The model under review builds one solid part; all positions refer to its coordinate system, in mm. A direction names the side the tool comes from. Round coordinates to 2 decimals unless told otherwise and drop trailing zeros. Loops run counter-clockwise (first coordinate to the right, second up) from the corner with the lowest first, then second, coordinate; pieces in that order, holes last. Notation, with made-up numbers: M 28,-35 L 76,-35 A14 cw 76,-19 Z; hole C 63,60.25 d8. An arc over 180 degrees is marked long. Use a Markdown table: item, result. Add a question column.
```python
from build123d import *

# Parameters (mm, degrees)
SKETCH_1_W          = 106
SKETCH_1_H          = 40
EXTRUDE_1_DEPTH     = 3
CUT_EXTRUDE_1_REACH = 58.727
SKETCH_2_R          = 4.25
SKETCH_2_R_2        = 2.75
CUT_EXTRUDE_2_REACH = 58.727
CUT_EXTRUDE_3_REACH = 58.727
SKETCH_4_W          = 2
SKETCH_4_H          = 4


with BuildPart() as part:
    # 草图1 → 凸台-拉伸1 (new body)
    with BuildSketch(Plane(origin=(0, 0, 0), x_dir=(1, 0, 0), z_dir=(0, 1, 0))):
        Rectangle(SKETCH_1_W, SKETCH_1_H)
    extrude(amount=EXTRUDE_1_DEPTH)

    # 草图2 → 切除-拉伸1 (cut, up to next)
    with BuildSketch(Plane(origin=(0, 3, 0), x_dir=(1, 0, 0), z_dir=(0, 1, 0)), mode=Mode.PRIVATE) as cut_extrude_1_sk1:
        with Locations(Location((-31.5, 0, 0), (0, 0, 270))):
            Circle(SKETCH_2_R)
    cut_extrude_1_tool1 = extrude(cut_extrude_1_sk1.sketch, amount=-CUT_EXTRUDE_1_REACH, mode=Mode.PRIVATE) & part.part
    # 草图2 → 切除-拉伸1 (cut, up to next)
    with BuildSketch(Plane(origin=(0, 3, 0), x_dir=(1, 0, 0), z_dir=(0, 1, 0)), mode=Mode.PRIVATE) as cut_extrude_1_sk2:
        with Locations(Location((31.5, 0, 0), (0, 0, 270))):
            Circle(SKETCH_2_R)
    cut_extrude_1_tool2 = extrude(cut_extrude_1_sk2.sketch, amount=-CUT_EXTRUDE_1_REACH, mode=Mode.PRIVATE) & part.part
    # 草图2 → 切除-拉伸1 (cut, up to next)
    with BuildSketch(Plane(origin=(0, 3, 0), x_dir=(1, 0, 0), z_dir=(0, 1, 0)), mode=Mode.PRIVATE) as cut_extrude_1_sk3:
        with Locations(Location((-47.5, 0, 0), (0, 0, 270))):
            Circle(SKETCH_2_R_2)
    cut_extrude_1_tool3 = extrude(cut_extrude_1_sk3.sketch, amount=-CUT_EXTRUDE_1_REACH, mode=Mode.PRIVATE) & part.part
    # 草图2 → 切除-拉伸1 (cut, up to next)
    with BuildSketch(Plane(origin=(0, 3, 0), x_dir=(1, 0, 0), z_dir=(0, 1, 0)), mode=Mode.PRIVATE) as cut_extrude_1_sk4:
        with Locations(Location((-15.5, 0, 0), (0, 0, 270))):
            Circle(SKETCH_2_R_2)
    cut_extrude_1_tool4 = extrude(cut_extrude_1_sk4.sketch, amount=-CUT_EXTRUDE_1_REACH, mode=Mode.PRIVATE) & part.part
    # 草图2 → 切除-拉伸1 (cut, up to next)
    with BuildSketch(Plane(origin=(0, 3, 0), x_dir=(1, 0, 0), z_dir=(0, 1, 0)), mode=Mode.PRIVATE) as cut_extrude_1_sk5:
        with Locations(Location((15.5, 0, 0), (0, 0, 270))):
            Circle(SKETCH_2_R_2)
    cut_extrude_1_tool5 = extrude(cut_extrude_1_sk5.sketch, amount=-CUT_EXTRUDE_1_REACH, mode=Mode.PRIVATE) & part.part
    # 草图2 → 切除-拉伸1 (cut, up to next)
    with BuildSketch(Plane(origin=(0, 3, 0), x_dir=(1, 0, 0), z_dir=(0, 1, 0)), mode=Mode.PRIVATE) as cut_extrude_1_sk6:
        with Locations(Location((47.5, 0, 0), (0, 0, 270))):
            Circle(SKETCH_2_R_2)
    cut_extrude_1_tool6 = extrude(cut_extrude_1_sk6.sketch, amount=-CUT_EXTRUDE_1_REACH, mode=Mode.PRIVATE) & part.part
    add(cut_extrude_1_tool1.solids().sort_by_distance((-31.5, 3, 0))[0], mode=Mode.SUBTRACT)
    add(cut_extrude_1_tool2.solids().sort_by_distance((31.5, 3, 0))[0], mode=Mode.SUBTRACT)
    add(cut_extrude_1_tool3.solids().sort_by_distance((-47.5, 3, 0))[0], mode=Mode.SUBTRACT)
    add(cut_extrude_1_tool4.solids().sort_by_distance((-15.5, 3, 0))[0], mode=Mode.SUBTRACT)
    add(cut_extrude_1_tool5.solids().sort_by_distance((15.5, 3, 0))[0], mode=Mode.SUBTRACT)
    add(cut_extrude_1_tool6.solids().sort_by_distance((47.5, 3, 0))[0], mode=Mode.SUBTRACT)

    # 草图3 → 切除-拉伸2 (cut, up to next)
    with BuildSketch(Plane(origin=(0, 3, 0), x_dir=(1, 0, 0), z_dir=(0, 1, 0)), mode=Mode.PRIVATE) as cut_extrude_2_sk1:
        Polygon((1.25, 13.25), (10, 13.25), (10, 3.75), (1.25, 3.75), (1.25, -8.75), (-1.25, -8.75), (-1.25, 3.75), (-10, 3.75), (-10, 13.25), (-1.25, 13.25), (-1.25, 17.25), (1.25, 17.25), align=None)
    cut_extrude_2_tool1 = extrude(cut_extrude_2_sk1.sketch, amount=-CUT_EXTRUDE_2_REACH, mode=Mode.PRIVATE) & part.part
    add(cut_extrude_2_tool1.solids().sort_by_distance((0, 3, -7.305405))[0], mode=Mode.SUBTRACT)

    # 草图4 → 切除-拉伸3 (cut, up to next)
    with BuildSketch(Plane(origin=(0, 3, 0), x_dir=(1, 0, 0), z_dir=(0, 1, 0)), mode=Mode.PRIVATE) as cut_extrude_3_sk1:
        with Locations((-3.75, 15.25)):
            Rectangle(SKETCH_4_W, SKETCH_4_H)
    cut_extrude_3_tool1 = extrude(cut_extrude_3_sk1.sketch, amount=-CUT_EXTRUDE_3_REACH, mode=Mode.PRIVATE) & part.part
    # 草图4 → 切除-拉伸3 (cut, up to next)
    with BuildSketch(Plane(origin=(0, 3, 0), x_dir=(1, 0, 0), z_dir=(0, 1, 0)), mode=Mode.PRIVATE) as cut_extrude_3_sk2:
        with Locations((3.75, 15.25)):
            Rectangle(SKETCH_4_W, SKETCH_4_H)
    cut_extrude_3_tool2 = extrude(cut_extrude_3_sk2.sketch, amount=-CUT_EXTRUDE_3_REACH, mode=Mode.PRIVATE) & part.part
    # 草图4 → 切除-拉伸3 (cut, up to next)
    with BuildSketch(Plane(origin=(0, 3, 0), x_dir=(1, 0, 0), z_dir=(0, 1, 0)), mode=Mode.PRIVATE) as cut_extrude_3_sk3:
        with Locations((3.75, -2.5)):
            Rectangle(SKETCH_4_W, SKETCH_4_H)
    cut_extrude_3_tool3 = extrude(cut_extrude_3_sk3.sketch, amount=-CUT_EXTRUDE_3_REACH, mode=Mode.PRIVATE) & part.part
    # 草图4 → 切除-拉伸3 (cut, up to next)
    with BuildSketch(Plane(origin=(0, 3, 0), x_dir=(1, 0, 0), z_dir=(0, 1, 0)), mode=Mode.PRIVATE) as cut_extrude_3_sk4:
        with Locations((-3.75, -2.5)):
            Rectangle(SKETCH_4_W, SKETCH_4_H)
    cut_extrude_3_tool4 = extrude(cut_extrude_3_sk4.sketch, amount=-CUT_EXTRUDE_3_REACH, mode=Mode.PRIVATE) & part.part
    add(cut_extrude_3_tool1.solids().sort_by_distance((-3.75, 3, -15.25))[0], mode=Mode.SUBTRACT)
    add(cut_extrude_3_tool2.solids().sort_by_distance((3.75, 3, -15.25))[0], mode=Mode.SUBTRACT)
    add(cut_extrude_3_tool3.solids().sort_by_distance((3.75, 3, 2.5))[0], mode=Mode.SUBTRACT)
    add(cut_extrude_3_tool4.solids().sort_by_distance((-3.75, 3, 2.5))[0], mode=Mode.SUBTRACT)


solid = part.part
```
(1) Consider section A-A, the plane x = -7.5. Give the boundary of the cut face in (y, z).
(2) Insertion check: pin 1 Ø13.5 at (x, z) = (-31.5, 0) entering from -Y; pin 2 Ø3.5 at (x, z) = (47.5, 0) entering from -Y. Each pin has a flat end and moves straight along its axis. Give the tip position at first contact, or say it passes through.
(3) Consider section C-C, the plane y = 1.3. Give the number of separate pieces and of enclosed holes in the cut face, then the cut area to 3 significant figures.
(4) Consider section B-B, the plane z = -11. Give the boundary of the cut face in (x, y).
(5) Draft analysis for pull direction X (two halves, no side actions). For faces 3 (the face through (0, 2, 8.75)), 4 (the face through (-53, 1, 0)), 5 (the face through (-1, 1, -20)), state which applies: released by +X, released by -X, zero draft, split by the parting line, or undercut.
(6) To check wall thickness, follow probe 1 along X at (y, z) = (2.95, -16); probe 2 along X at (y, z) = (1.9, -12.5); probe 3 along Z at (x, y) = (-8, 1.35). State the ranges of each line that lie inside material, in increasing order.
(7) For faces 1 (the face through (7, 2, -13.25)), 2 (the face through (-1, 1, 20)), list the 3-axis set-ups (+Z, -Z, +X, -X, +Y, -Y) from which the entire face can be reached by the end or side of a thin tool; tool diameter is ignored.
Found:
| question | item | result |
|---|---|---|
| 1 | outline | M 0,-20 L 3,-20 L 3,-13.25 L 0,-13.25 Z; M 0,-3.75 L 3,-3.75 L 3,20 L 0,20 Z |
| 2 | pin 1 | stops at y = 0 |
| 2 | pin 2 | passes through |
| 3 | separate pieces | 1 |
| 3 | enclosed holes | 9 |
| 3 | area | 3,770 mm^2 |
| 4 | outline | M -53,0 L -10,0 L -10,3 L -53,3 Z; M 10,0 L 53,0 L 53,3 L 10,3 Z |
| 5 | face 3 | undercut |
| 5 | face 4 | released by -X |
| 5 | face 5 | zero draft |
| 6 | probe 1 | x = -53 to -4.75, -2.75 to -1.25, 1.25 to 2.75, 4.75 to 53 |
| 6 | probe 2 | x = -53 to -10, 10 to 53 |
| 6 | probe 3 | z = -20 to -13.25, -3.75 to 20 |
| 7 | face 1 | +Y, -Y |
| 7 | face 2 | +Z, +X, -X, +Y, -Y |
